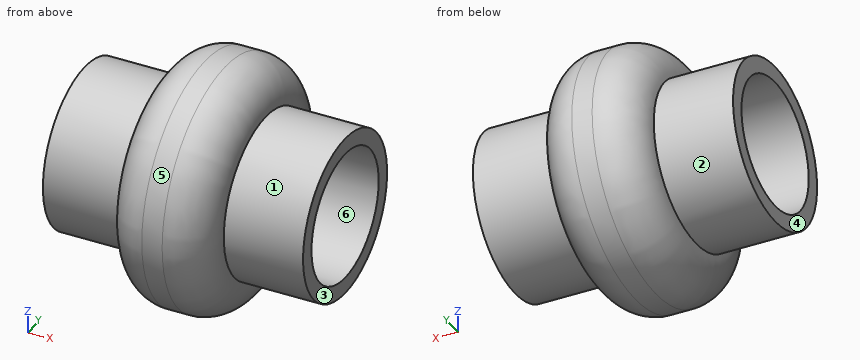
from build123d import *

# Parameters (mm, degrees)
SKETCH1_R           = 3
BOSS_EXTRUDE1_DEPTH = 1.25
SKETCH2_R           = 2
BOSS_EXTRUDE2_DEPTH = 1.95
BOSS_EXTRUDE8_START = 1.95
SKETCH3_R           = 2
BOSS_EXTRUDE8_DEPTH = 1.95
SKETCH4_R           = 1.6
CUT_EXTRUDE1_DEPTH  = 8.678541528
FILLET1_R           = 1


with BuildPart() as part:
    # Sketch1 → Boss-Extrude1 (new, symmetric)
    with BuildSketch(Plane(origin=(0, 0, 0), x_dir=(0, 0, -1), z_dir=(1, 0, 0))):
        Circle(SKETCH1_R)
    extrude(amount=BOSS_EXTRUDE1_DEPTH, both=True)

    # Sketch2 → Boss-Extrude2 (add)
    with BuildSketch(Plane(origin=(1.25, 0, 0), x_dir=(0, 0, -1), z_dir=(1, 0, 0))):
        Circle(SKETCH2_R)
    extrude(amount=BOSS_EXTRUDE2_DEPTH)

    # Sketch3 → Boss-Extrude8 (add)
    with BuildSketch(Plane.ZY.offset(1.25).offset(BOSS_EXTRUDE8_START)):
        with Locations(Location((0, 0, 0), (0, 0, 180))):
            Circle(SKETCH3_R)
    extrude(amount=-BOSS_EXTRUDE8_DEPTH)

    # Sketch4 → Cut-Extrude1 (cut, through all)
    with BuildSketch(Plane(origin=(3.2, 0, 0), x_dir=(0, 0, -1), z_dir=(1, 0, 0))):
        Circle(SKETCH4_R)
    extrude(amount=-CUT_EXTRUDE1_DEPTH, mode=Mode.SUBTRACT)

    # Fillet1
    fillet1_edges = [part.edges().sort_by_distance(p)[0] for p in [
        (-1.25, 0, 3),
        (1.25, 0, 3),
    ]]
    fillet(fillet1_edges, radius=FILLET1_R - 0.0001)  # a hair under: the kernel refuses the full size


solid = part.part
Model file for the job. Use its own axes, mm. Face numbers are marked on the shaded views. A direction names the side the tool comes from. Give positions to 0.01 mm unless a question says otherwise; leave off trailing zeros. Order: outer loops, then holes, each group sorted by start corner. A loop starts at its lowest first (then second) coordinate and runs counter-clockwise, first axis right, second up. Notation, with made-up numbers: (70.25, -10.5) - (74.25, -10.5) arc R30 cw to (74.25, 12.5) - close; hole circle Ø2 at (-1, 24.25). An arc over 180 degrees is marked (long way). Return JSON: item names as keys, results as strings.
1) 3-axis set-ups, long thin cutter, end or side, ignore diameter. For the marked faces 1, 2 and 3: which of +Z, -Z, +X, -X, +Y, -Y reach the whole face in a straight line?
Geometry says:
{"face 1": "+X", "face 2": "-X", "face 3": "+Z, -Z, +X, +Y, -Y"}
2) Probe line 1 (Y direction, x = 1.5, z = 0); line 2 (X direction, y = -1, z = 1.8); line 3 (Y direction, x = -1.5, z = 1.1). List the from-to ranges inside material, lowest first. Write a range as from..to.
Geometry says:
{"line 1": "-2..-1.6, 1.6..2", "line 2": "-1.25..1.25", "line 3": "-1.67..-1.16, 1.16..1.67"}
3) Pull direction Y, two halves, no side cores. Call the marked faces 4, 5 and 6: pulls with the +Y half, pulls with the -Y half, needs draft (parallel to the pull), parting line crosses it, or undercut.
Geometry says:
{"face 4": "needs draft", "face 5": "parting line crosses it", "face 6": "undercut"}
4) Cut at C-C, the plane x = 2.5. Give the cut face in (y, z).
Geometry says:
{"outline": "circle Ø4 at (0, 0); hole circle Ø3.2 at (0, 0)"}
5) Flat gauge pin, fed straight in: P1, Ø2, axis at x = 0.5, y = 2.5, coming from the -Z side. Where does the tip first touch, or does it go through?
Geometry says:
{"P1": "z = -2.59"}
6) Cut at D-D, the plane x = 1. Give the cut face in (y, z), plus the area to 3 significant figures.
Geometry says:
{"outline": "circle Ø5.32 at (0, 0); hole circle Ø3.2 at (0, 0)", "area": "14.2 mm²"}
